Part model, mm, in its own coordinate system. A direction names the side the tool comes from. Give positions to 0.01 mm unless a question says otherwise; leave off trailing zeros. Order: outer loops, then holes, each group sorted by start corner. A loop starts at its lowest first (then second) coordinate and runs counter-clockwise, first axis right, second up.
1. Probe line 1 (Y direction, x = 191, z = -5.25); line 2 (X direction, y = -140, z = -6.75); line 3 (Z direction, x = 212, y = -181). List the from-to ranges inside material, lowest first.
2. Slice it at B-B on x = 269. List the corners of the cut face in (y, z).
3. Slice it at C-C on y = -145.5. List the corners of the cut face in (x, z), and give its area (3 significant figures).
4. Slice it at A-A on z = -3. List the corners of the cut face in (x, y), and give its area (3 significant figures).
5. Drop a flat-ended pin along its axis: pin 1 Ø10 at (x, y) = (211.5, -162.5) entering from +Z. Give the stop position or say it passes through.
6. Which spindle directions (+Z, -Z, +X, -X, +Y, -Y) get a long thin tool onto all of the face, cutting with end or side? Do faces 4 (the flat face through (322.541, -139, -5)), 5 (the flat face through (245, -137, -7)). Say none if no direction does.
7. Mould opens along Y. For faces 1 (the cylindrical face through (318.55, -63.43, -4.93)), 2 (the flat face through (246, -62, 0)), 3 (the flat face through (319.341, -139, -3)) say: +Y half, -Y half, draft (parallel to the pull), parting line (faces both ways), or undercut.
Autodesk Inventor part; units mm, degrees
ref_plane "YZ Plane" through (0, 0, 0) normal (1, 0, 0) x (0, 1, 0)
ref_plane "XZ Plane" through (0, 0, 0) normal (0, 1, 0) x (-1, 0, 0)
ref_plane "XY Plane" through (0, 0, 0) normal (0, 0, 1) x (1, 0, 0)
ref_plane "Work Plane2" through (0, 0, 0) normal (0, 0, 1) x (1, 0, 0)
sketch "Sketch2" plane through (0, 0, 0) normal (0, 0, 1) x (1, 0, 0)
  line L0 (174.2186, -202.7504) -> (174.2186, -73.2206)
  arc A0 (184.2186, -63.2206) -> (174.2186, -73.2206) centre (184.2186, -73.2206) ccw
  circle A1 centre (184.2186, -73.2206) radius 3
  line L1 (184.2186, -63.2206) -> (308.5414, -63.2206)
  circle A2 centre (308.5414, -73.2206) radius 3
  arc A3 (318.5414, -73.2206) -> (308.5414, -63.2206) centre (308.5414, -73.2206) ccw
  line L2 (318.5414, -73.2206) -> (318.5414, -202.7504)
  arc A4 (308.5414, -212.7504) -> (318.5414, -202.7504) centre (308.5414, -202.7504) ccw
  line L3 (308.5414, -212.7504) -> (184.2186, -212.7504)
  arc A5 (174.2186, -202.7504) -> (184.2186, -212.7504) centre (184.2186, -202.7504) ccw
  circle A6 centre (184.2186, -202.7504) radius 3
  circle A7 centre (308.5414, -202.7504) radius 3
  line L4 (308.5414, -59.2206) -> (184.2186, -59.2206)
  arc A8 (184.2186, -59.2206) -> (170.2186, -73.2206) centre (184.2186, -73.2206) ccw
  line L5 (170.2186, -73.2206) -> (170.2186, -202.7504)
  arc A9 (170.2186, -202.7504) -> (184.2186, -216.7504) centre (184.2186, -202.7504) ccw
  line L6 (184.2186, -216.7504) -> (308.5414, -216.7504)
  arc A10 (308.5414, -216.7504) -> (322.5414, -202.7504) centre (308.5414, -202.7504) ccw
  line L7 (322.5414, -202.7504) -> (322.5414, -73.2206)
  arc A11 (322.5414, -73.2206) -> (308.5414, -59.2206) centre (308.5414, -73.2206) ccw
  arc A12 (184.2186, -63.7206) -> (174.7186, -73.2206) centre (184.2186, -73.2206) ccw
  point P0 (0, 0)
  dimension "d8" = 4
ref_plane "Work Plane3" through (0, 0, 0) normal (0, 0, 1) x (1, 0, 0)
extrude "Extrusion3" add sketch "Sketch2" against normal blind 10 contours L0 A0 L1 A3 L2 A4 L3 A5 | A11 L7 A10 L6 A9 L5 A8 L4
sketch "Sketch4" plane through (0, 0, 0) normal (0, 0, 1) x (1, 0, 0)
  circle A0 centre (308.5414, -202.7504) radius 3
  circle A1 centre (184.2186, -202.7504) radius 3
  circle A2 centre (308.5414, -73.2206) radius 3
  circle A3 centre (184.2186, -73.2206) radius 3
  arc A4 (184.2186, -59.2206) -> (170.2186, -73.2206) centre (184.2186, -73.2206) ccw
  line L0 (170.2186, -73.2206) -> (170.2186, -202.7504)
  arc A5 (170.2186, -202.7504) -> (184.2186, -216.7504) centre (184.2186, -202.7504) ccw
  line L1 (184.2186, -216.7504) -> (308.5414, -216.7504)
  arc A6 (308.5414, -216.7504) -> (322.5414, -202.7504) centre (308.5414, -202.7504) ccw
  line L2 (322.5414, -202.7504) -> (322.5414, -73.2206)
  arc A7 (322.5414, -73.2206) -> (308.5414, -59.2206) centre (308.5414, -73.2206) ccw
  line L3 (308.5414, -59.2206) -> (184.2186, -59.2206)
  arc A8 (184.2186, -62.4206) -> (173.4186, -73.2206) centre (184.2186, -73.2206) ccw
  line L4 (173.4186, -73.2206) -> (173.4186, -202.7504)
  arc A9 (173.4186, -202.7504) -> (184.2186, -213.5504) centre (184.2186, -202.7504) ccw
  line L5 (184.2186, -213.5504) -> (308.5414, -213.5504)
  arc A10 (308.5414, -213.5504) -> (319.3414, -202.7504) centre (308.5414, -202.7504) ccw
  line L6 (319.3414, -202.7504) -> (319.3414, -73.2206)
  arc A11 (319.3414, -73.2206) -> (308.5414, -62.4206) centre (308.5414, -73.2206) ccw
  line L7 (308.5414, -62.4206) -> (184.2186, -62.4206)
  point P0 (0, 0)
  dimension "d10" = 3.2
extrude "Extrusion4" cut sketch "Sketch4" against normal blind 7 contours L7 A11 L6 A10 L5 A9 L4 A8
sketch "Sketch5" plane through (0, 0, -10) normal (0, 0, -1) x (-1, 0, 0)
  circle A0 centre (-308.5414, -202.7504) radius 3
  circle A1 centre (-184.2186, -202.7504) radius 3
  circle A2 centre (-308.5414, -73.2206) radius 3
  circle A3 centre (-184.2186, -73.2206) radius 3
  circle A4 centre (-308.5414, -73.2206) radius 2.5
  circle A5 centre (-184.2186, -73.2206) radius 2.5
  circle A6 centre (-184.2186, -202.7504) radius 2.5
  circle A7 centre (-308.5414, -202.7504) radius 2.5
  point P0 (0, 0)
  dimension "d15" = 0.5
  dimension "d16" = 0.5
  dimension "d17" = 0.5
  dimension "d18" = 0.5
extrude "Extrusion5" add sketch "Sketch5" against normal up to surface (3 mm away)
sketch "Sketch6" plane through (0, 0, -10) normal (0, 0, -1) x (-1, 0, 0)
  circle A0 centre (-184.2186, -202.7504) radius 2.5
  circle A1 centre (-308.5414, -73.2206) radius 2.5
  circle A2 centre (-308.5414, -202.7504) radius 2.5
  circle A3 centre (-184.2186, -73.2206) radius 2.5
  point P0 (0, 0)
extrude "Extrusion6" add sketch "Sketch6" against normal blind 20.75
properties part number "Part_atas"
Data:
1. line 1: y = -216.75 to -213.55, -62.42 to -59.22
1. line 2: x = 170.22 to 173.42, 319.34 to 322.54
1. line 3: z = -10 to -7
2. outline: (-216.75, -10) - (-59.22, -10) - (-59.22, 0) - (-62.42, 0) - (-62.42, -7) - (-213.55, -7) - (-213.55, 0) - (-216.75, 0) - close
3. outline: (170.22, -10) - (322.54, -10) - (322.54, 0) - (319.34, 0) - (319.34, -7) - (173.42, -7) - (173.42, 0) - (170.22, 0) - close
3. area: 502 mm2
4. outline: (170.22, -202.75) arc R14 ccw to (184.22, -216.75) - (308.54, -216.75) arc R14 ccw to (322.54, -202.75) - (322.54, -73.22) arc R14 ccw to (308.54, -59.22) - (184.22, -59.22) arc R14 ccw to (170.22, -73.22) - close; circle Ø5 at (184.22, -202.75); circle Ø5 at (184.22, -73.22); circle Ø5 at (308.54, -202.75); circle Ø5 at (308.54, -73.22); hole (173.42, -202.75) arc R10.8 ccw to (184.22, -213.55) - (308.54, -213.55) arc R10.8 ccw to (319.34, -202.75) - (319.34, -73.22) arc R10.8 ccw to (308.54, -62.42) - (184.22, -62.42) arc R10.8 ccw to (173.42, -73.22) - close
4. area: 1,950 mm2
5. pin 1: stops at z = -7
6. face 4: +Z, -Z, +X, +Y, -Y
6. face 5: +Z
7. face 1: +Y half
7. face 2: draft
7. face 3: undercut
